Autodesk Inventor part; units mm, degrees
ref_plane "YZ Plane" through (0, 0, 0) normal (1, 0, 0) x (0, 1, 0)
ref_plane "XZ Plane" through (0, 0, 0) normal (0, 1, 0) x (-1, 0, 0)
ref_plane "XY Plane" through (0, 0, 0) normal (0, 0, 1) x (1, 0, 0)
sketch "Эскиз1" plane through (0, 0, 0) normal (0, 1, 0) x (-1, 0, 0)
  line L0 (-6, -33) -> (6, -33)
  line L1 (6, -33) -> (6, 33)
  line L2 (6, 33) -> (-6, 33)
  line L3 (-6, 33) -> (-6, -33)
  line L4 (-6, -33) -> (6, 33) construction
  line L5 (6, -33) -> (-6, 33) construction
  circle A0 centre (-0.6, 0) radius 1.5
  point P0 (0, 0)
  dimension "d0" = 12
  dimension "d1" = 66
  dimension "d21" = 3
  dimension "d22" = 0.6
  dimension "d23" = 33
extrude "Выдавливание1" add sketch "Эскиз1" along normal blind 5
sketch "Эскиз2" plane through (0, 0, 0) normal (0, -1, 0) x (1, 0, 0)
  line L0 (-3, -33) -> (-8, -33)
  line L1 (-8, -33) -> (-8, -21)
  line L2 (-8, -21) -> (-3, -21)
  line L3 (-3, -21) -> (-3, -33) construction
  line L4 (-6, -33) -> (-6, 33)
  line L5 (6, -33) -> (-6, -33)
  line L6 (-6, 0) -> (6, 0) construction
  line L7 (6, 33) -> (6, -33)
  line L8 (0, -33) -> (0, 33) construction
  line L9 (-6, 33) -> (6, 33)
  line L10 (-3, 33) -> (-8, 33)
  line L11 (-8, 33) -> (-8, 21)
  line L12 (-8, 21) -> (-3, 21)
  line L13 (-3, 21) -> (-3, 33) construction
  line L14 (3, -33) -> (8, -33)
  line L15 (8, -33) -> (8, -21)
  line L16 (8, -21) -> (3, -21)
  line L17 (3, -21) -> (3, -33) construction
  line L18 (8, 21) -> (3, 21)
  line L19 (8, 33) -> (8, 21)
  line L20 (3, 33) -> (8, 33)
  line L21 (3, 21) -> (3, 33) construction
  line L22 (-3, -33) -> (3, -33)
  line L23 (-3, -21) -> (3, -21)
  line L24 (-3, 21) -> (3, 21)
  line L25 (-3, 33) -> (3, 33)
  point P0 (0, 0)
  dimension "d5" = 2
  dimension "d6" = 5
  dimension "d7" = 12
  dimension "d8" = 0
extrude "Выдавливание2" add sketch "Эскиз2" along normal blind 15 and the other way blind 5 contours L0 L4 L2 L23 L16 L7 L5 | L0 L1 L2 L4 | L7 L16 L15 L14 | L12 L11 L10 L4 | L4 L9 L7 L18 L24 L12 | L7 L20 L19 L18
fillet "Сопряжение1" radius 1 8 edges at (-8, -5, -21) (-8, -5, 33) (-8, -5, 21) (8, -5, -21) (8, -5, -33) (-8, -5, -33) (8, -5, 33) (8, -5, 21)
sketch "Эскиз3" plane through (0, 5, 0) normal (0, 1, 0) x (1, 0, 0)
  circle A0 centre (0.6, 0) radius 1.5
  circle A1 centre (0.6, 0) radius 4.5
  point P0 (0, 0)
  dimension "d24" = 9
extrude "Выдавливание3" cut sketch "Эскиз3" against normal blind 2.5
sketch "Эскиз4" plane through (0, -15, 0) normal (0, -1, 0) x (1, 0, 0)
  arc A0 (-7, -21) -> (-8, -22) centre (-7, -22) ccw
  arc A1 (7, -33) -> (8, -32) centre (7, -32) ccw
  line L0 (-7, -22) -> (7, -32) construction
  circle A2 centre (0, -27) radius 3
  line L1 (0, 0) -> (-6, 0) construction
  line L2 (-6, -21) -> (-6, 21)
  circle A3 centre (0, 27) radius 3
  dimension "d18" = 6
extrude "Выдавливание4" cut sketch "Эскиз4" against normal blind 15
equation "\"d23\" = 0.5 * d1"
properties part number "kick"
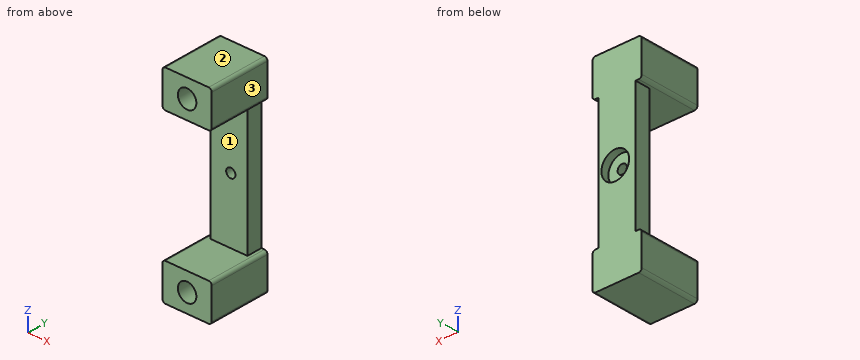
The listing builds one solid part. Answer for the finished solid, in the listing's coordinates (mm). Face numbers are marked on the shaded views. Give positions to 0.01 mm unless a question says otherwise; leave off trailing zeros. Loops run counter-clockwise (first coordinate to the right, second up) from the corner with the lowest first, then second, coordinate; pieces in that order, holes last. Notation, with made-up numbers: M 54,27 L 65,27 A29 cw 65,58 Z; hole C 65,-38 d8. An arc over 180 degrees is marked long. Answer as CSV lines item,"result".
Item 1: The part is cut by section B-B (z = 0). Give the vertices of the cut face in (x, y).
Values follow:
outline,"M -6,0 L -0.9,0 L -0.9,2.5 L -3.9,2.5 L -3.9,5 L -6,5 Z; M 2.1,0 L 6,0 L 6,5 L 5.1,5 L 5.1,2.5 L 2.1,2.5 Z"
Item 2: The part is cut by section D-D (z = 27). Give the vertices of the cut face in (x, y), and give its area (3 significant figures).
Values follow:
outline,"M -8,-15 L -3,-15 L -3,0 L 3,0 L 3,-15 L 8,-15 L 8,5 L -8,5 Z"
area,"230 mm^2"
Item 3: The part is cut by section C-C (x = 0). Give the vertices of the cut face in (y, z).
Values follow:
outline,"M -15,-33 L 5,-33 L 5,-4.46 L 2.5,-4.46 L 2.5,-1.37 L 0,-1.37 L 0,-21 L -15,-21 L -15,-24 L 0,-24 L 0,-30 L -15,-30 Z; M -15,21 L 0,21 L 0,1.37 L 2.5,1.37 L 2.5,4.46 L 5,4.46 L 5,33 L -15,33 L -15,30 L 0,30 L 0,24 L -15,24 Z"
Item 4: Given pin 1 Ø1 at (x, z) = (1.5, 19) entering from -Y; pin 2 Ø1.5 at (y, z) = (3, -6) entering from -X; pin 3 Ø2.5 at (y, z) = (3, -7) entering from +X, each flat-ended and moving along its own axis, determine where each tip first touches the part or whether it passes through.
Values follow:
pin 1,"stops at y = 0"
pin 2,"stops at x = -6"
pin 3,"stops at x = 6"
Item 5: The mould has two halves that part along Z. Classify the marked faces 1, 2 and 3: released by +Z, released by -Z, zero draft, split by the parting line, or undercut.
Values follow:
face 1,"undercut"
face 2,"released by +Z"
face 3,"zero draft"
Item 6: Straight lines are drawn through the part: line 1 along Z through (x, y) = (0, -10.75); line 2 along Z through (x, y) = (-4.25, -8.75); line 3 along Z through (x, y) = (0.6, 3.3). For each, find the intervals that lie inside material, in ascending order. Write a range as [from, to].
Values follow:
line 1,"z = [-33, -30], [-24, -21], [21, 24], [30, 33]"
line 2,"z = [-33, -21], [21, 33]"
line 3,"z = [-33, -4.5], [4.5, 33]"
Item 7: The part is cut by section A-A (y = -7). Give the vertices of the cut face in (x, z), and give its area (3 significant figures).
Values follow:
outline,"M -8,-32 A1 ccw -7,-33 L 7,-33 A1 ccw 8,-32 L 8,-22 A1 ccw 7,-21 L -7,-21 A1 ccw -8,-22 Z; M -8,22 A1 ccw -7,21 L 7,21 A1 ccw 8,22 L 8,32 A1 ccw 7,33 L -7,33 A1 ccw -8,32 Z; hole C 0,-27 d6; hole C 0,27 d6"
area,"326 mm^2"
